from build123d import *
from build123d.topology import SkipClean

# Parameters (mm, degrees)
EXTRUDE_1_DEPTH     = 2
EXTRUDE_2_DEPTH     = 13
SKETCH_4_R          = 1.5
CUT_EXTRUDE_1_DEPTH = 27.046428912
SKETCH_5_R          = 1.5
CUT_EXTRUDE_2_DEPTH = 27.046428912


with BuildPart() as part:
    # 草图1 → 凸台-拉伸1 (new body)
    with BuildSketch(Plane(origin=(0, 0, 0), x_dir=(1, 0, 0), z_dir=(0, 1, 0))):
        with BuildLine():
            Line((-15.918812675, 3), (18.081187325, 3))
            ThreePointArc((18.081187325, 3), (21.081187325, 0), (18.081187325, -3))
            Line((18.081187325, -3), (-15.918812675, -3))
            ThreePointArc((-15.918812675, -3), (-18.918812675, 0), (-15.918812675, 3))
        make_face()
    extrude(amount=EXTRUDE_1_DEPTH)

    # 草图2 → 凸台-拉伸2 (add)
    with SkipClean():  # the faces are left unmerged after this step: merging them gives an invalid solid
        with BuildSketch(Plane(origin=(0, 2, 0), x_dir=(1, 0, 0), z_dir=(0, 1, 0))):
            with BuildLine():
                ThreePointArc((-15.918812675, 3), (-18.918812675, 0), (-15.918812675, -3))
                ThreePointArc((-15.918812675, -3), (-13.797492331, -2.121320344), (-12.918812675, 0))
                ThreePointArc((-12.918812675, 0), (-13.797492331, 2.121320344), (-15.918812675, 3))
            make_face()
            with BuildLine():
                ThreePointArc((18.081187325, 3), (15.081187325, 0), (18.081187325, -3))
                ThreePointArc((18.081187325, -3), (20.202507669, -2.121320344), (21.081187325, 0))
                ThreePointArc((21.081187325, 0), (20.202507669, 2.121320344), (18.081187325, 3))
            make_face()
        extrude(amount=EXTRUDE_2_DEPTH)

    # 草图4 → 切除-拉伸1 (cut, through all)
    with SkipClean():  # the faces are left unmerged after this step: merging them gives an invalid solid
        with BuildSketch(Plane(origin=(0, 15, 0), x_dir=(1, 0, 0), z_dir=(0, 1, 0))):
            with Locations(Location((-15.918812675, 0, 0), (0, 0, 270))):
                Circle(SKETCH_4_R)
        extrude(amount=-CUT_EXTRUDE_1_DEPTH, mode=Mode.SUBTRACT)

    # 草图5 → 切除-拉伸2 (cut, through all)
    with SkipClean():  # the faces are left unmerged after this step: merging them gives an invalid solid
        with BuildSketch(Plane(origin=(0, 15, 0), x_dir=(1, 0, 0), z_dir=(0, 1, 0))):
            with Locations(Location((18.081187325, 0, 0), (0, 0, 270))):
                Circle(SKETCH_5_R)
        extrude(amount=-CUT_EXTRUDE_2_DEPTH, mode=Mode.SUBTRACT)


solid = part.part
Verification items for the finished model (mm, model axes). Coordinates: 2 decimals unless noted, no trailing zeros. Order: outer loops, then holes, each group sorted by start corner. A loop starts at its lowest first (then second) coordinate and runs counter-clockwise, first axis right, second up.
1. Release check for a two-part mould opening along Z. For faces 1 (the face through (1, 1, 3)), 2 (the face through (19.4, 15, 1.3)), 3 (the face through (1, 1, -3)), 4 (the face through (-17.383, 7.605, -0.325)) record: +Z half, -Z half, draft (parallel to the pull), parting line (faces both ways), or undercut.
Results found:
face 1: +Z half
face 2: draft
face 3: -Z half
face 4: undercut
2. Sectioned sample at A-A, the plane y = 6.75. Record the cut outline in (x, z).
Results found:
outline: circle Ø6 at (-15.92, 0); circle Ø6 at (18.08, 0); hole circle Ø3 at (-15.92, 0); hole circle Ø3 at (18.08, 0)
3. Sectioned sample at B-B, the plane z = -1. Record the cut outline in (x, y).
Results found:
outline: (-18.75, 0) - (-17.04, 0) - (-17.04, 15) - (-18.75, 15) - close; (-14.8, 0) - (16.96, 0) - (16.96, 15) - (15.25, 15) - (15.25, 2) - (-13.09, 2) - (-13.09, 15) - (-14.8, 15) - close; (19.2, 0) - (20.91, 0) - (20.91, 15) - (19.2, 15) - close
4. Sectioned sample at C-C, the plane x = 4. Record the cut outline in (y, z).
Results found:
outline: (0, -3) - (2, -3) - (2, 3) - (0, 3) - close
5. Go/stop test with flat-tipped pins: pin 1 Ø1 at (y, z) = (8.5, 2.5) entering from +X; pin 2 Ø2.5 at (x, z) = (-15.92, 0) entering from +Y. Record where each tip stops, or that it passes through.
Results found:
pin 1: stops at x = 20.32
pin 2: passes through
6. Sectioned sample at D-D, the plane z = 0.75. Record the cut outline in (x, y).
Results found:
outline: (-18.82, 0) - (-17.22, 0) - (-17.22, 15) - (-18.82, 15) - close; (-14.62, 0) - (16.78, 0) - (16.78, 15) - (15.18, 15) - (15.18, 2) - (-13.01, 2) - (-13.01, 15) - (-14.62, 15) - close; (19.38, 0) - (20.99, 0) - (20.99, 15) - (19.38, 15) - close
7. Scan lines: line 1 (X direction, y = 4.25, z = 0); line 2 (X direction, y = 6, z = -1); line 3 (Z direction, x = 17, y = 5). Record each from-to range of solid material in increasing order.
Results found:
line 1: x = -18.92 to -17.42, -14.42 to -12.92, 15.08 to 16.58, 19.58 to 21.08
line 2: x = -18.75 to -17.04, -14.8 to -13.09, 15.25 to 16.96, 19.2 to 20.91
line 3: z = -2.8 to -1.04, 1.04 to 2.8
